For this review, take the finished solid that the model builds, in its own axes (mm). Face numbers are marked on the shaded views. A direction names the side the tool comes from. Give positions to 0.01 mm unless a question says otherwise; leave off trailing zeros. Write each loop counter-clockwise with the first axis right and the second up, starting at its lowest first coordinate (ties: lowest second). Pieces come first, ordered by that corner, then holes. Notation, with made-up numbers: M -34,54.25 L -14,54.25 A27 ccw -14,72.25 Z; hole C 24.5,-29.5 d11. An arc over 180 degrees is marked long. Use one line per item in the form item = value. Start each with the question number.
Q1. For probe 1 along Y at (x, z) = (28, 2.25); probe 2 along X at (y, z) = (-0.75, 10.75); probe 3 along Z at (x, y) = (10, -5.75), list the stretches that pass through material, from the lowest coordinate up. Write a range as [from, to].
Q2. Clearance check with flat-ended pins moving along their axes: pin 1 Ø4.5 at (x, z) = (7.5, 6.5) entering from -Y; pin 2 Ø1 at (y, z) = (-3.5, 10) entering from +X; pin 3 Ø3 at (y, z) = (-4.5, 2) entering from -X; pin 4 Ø4.5 at (x, y) = (-13.24, -3.03) entering from -Z. State where each tip first meets the part, or that it passes through.
Q3. Consider section B-B on z = 4. Write out the cut boundary in (x, y), and give its area (3 significant figures).
Q4. Tool access review of the marked faces 1 and 2: name each direction out of +Z, -Z, +X, -X, +Y, -Y from which nothing blocks a thin tool from reaching the whole face with its end or side.
Q5. Consider section A-A on x = -57. Write out the cut boundary in (y, z).
```python
from build123d import *

# Parameters (mm, degrees)
F0_W      = 34
F0_H      = 10
F1_DEPTH  = 11
F2_W      = 2.5
F2_H      = 11
F3_DEPTH  = 58
F4_W      = 2.5
F4_H      = 11
F5_DEPTH  = 58
F6_W      = 7.5
F6_H      = 9
F7_DEPTH  = 92.001
F8_R      = 1.85
F9_DEPTH  = 2.001
F10_R     = 1
F11_W     = 150
F11_H     = 2
F12_DEPTH = 1.5
F13_R     = 1.99999


# Not quite as in the source:
# - a fillet or chamfer is up to 0.001 mm smaller than in the source, because OpenCascade refuses the exact size


with BuildPart() as f1:
    # F0 (on Top) → F1 (new body)
    with BuildSketch(Plane.XY):
        with Locations((-3.2397536635, -4.5336725935)):
            Rectangle(F0_W, F0_H)
    extrude(amount=F1_DEPTH)

    # F2 (on face) → F3 (join)
    with BuildSketch(Plane(origin=(-20.2397536635, 0, 0), x_dir=(0, -1, 0), z_dir=(-1, 0, 0))):
        with Locations((8.2836725935, 5.5)):
            Rectangle(F2_W, F2_H)
    extrude(amount=F3_DEPTH)

    # F4 (on face) → F5 (join)
    with BuildSketch(Plane.YZ.offset(13.7602463365)):
        with Locations((-8.2836725935, 5.5)):
            Rectangle(F4_W, F4_H)
    extrude(amount=F5_DEPTH)

    # F6 (on face) → F7 (cut, through all)
    with BuildSketch(Plane.YZ.offset(13.7602463365)):
        with Locations((-3.2836725935, 4.5)):
            Rectangle(F6_W, F6_H)
    extrude(amount=-F7_DEPTH, mode=Mode.SUBTRACT)

    # F8 (on face) → F9 (cut, through all)
    with BuildSketch(Plane(origin=(0, 0, 9), x_dir=(1, 0, 0), z_dir=(0, 0, -1))):
        with Locations((-13.2397536635, 3.0336725935)):
            Circle(F8_R)
        with Locations((6.7602463365, 3.0336725935)):
            Circle(F8_R)
    extrude(amount=-F9_DEPTH, mode=Mode.SUBTRACT)

    # F10
    f10_edges = [f1.edges().sort_by_distance(p)[0] for p in [
        (-3.239754, -7.033673, 9),
        (-20.239754, -7.033673, 10),
        (13.760246, -7.033673, 10),
        (-20.239754, 0.466327, 10),
        (13.760246, 0.466327, 10),
    ]]
    fillet(f10_edges, radius=F10_R)

    # F11 (on face) → F12 (join)
    with BuildSketch(Plane.XZ.offset(9.5336725935)):
        with Locations((-3.2397536635, 10)):
            Rectangle(F11_W, F11_H)
    extrude(amount=F12_DEPTH)

    # F13 (radius 2 in the source; OpenCascade refuses exactly that, so slightly less here)
    f13_edges = [f1.edges().sort_by_distance(p)[0] for p in [
        (-78.239754, -9.033673, 11),
        (-78.239754, -8.283673, 0),
        (71.760246, -9.033673, 11),
        (71.760246, -8.283673, 0),
    ]]
    fillet(f13_edges, radius=F13_R)


solid = f1.part
```
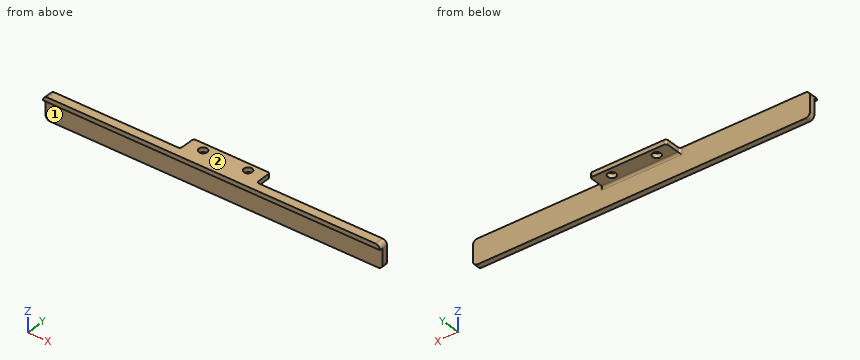
Working result:
q1.probe_1 = [-9.53, -7.03]
q1.probe_2 = [-20.24, 13.76]
q1.probe_3 = [9, 11]
q2.pin_1 = -9.53
q2.pin_2 = 13.76
q2.pin_3 = through
q2.pin_4 = 9
q3.outline = M -78.24,-9.53 L 71.76,-9.53 L 71.76,-7.03 L -78.24,-7.03 Z
q3.area = 375 mm²
q4.face_1 = -Z, +X, -X, -Y
q4.face_2 = +Z, +X, -X, +Y, -Y
q5.outline = M -11.03,9 L -9.53,9 L -9.53,0 L -7.03,0 L -7.03,11 L -11.03,11 Z
